Read the model definition and answer for the solid it produces. Units are mm, in the model's axes. Face numbers are marked on the shaded views. A direction names the side the tool comes from. Give positions to 0.01 mm unless a question says otherwise; leave off trailing zeros. Write each loop counter-clockwise with the first axis right and the second up, starting at its lowest first coordinate (ties: lowest second). Pieces come first, ordered by that corner, then holes. Notation, with made-up numbers: (-5, 43) -> (28, 43) arc R9 cw to (28, 49) -> close; hole circle Ø3 at (-32, 56.5). An arc over 180 degrees is marked (long way). Write item = value, one per line.
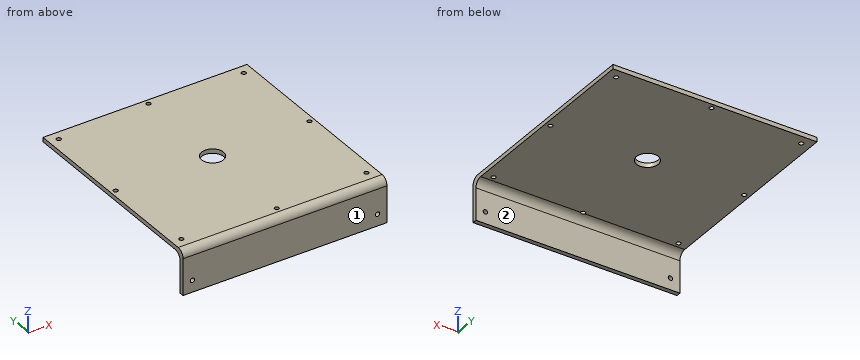
from build123d import *

# Parameters (mm, degrees)
SKICA1_W                 = 140
SKICA1_H                 = 145
SKICA1_R                 = 1.5
P_IDAT_VYSUNUT_M1_DEPTH  = 3
SKICA2_W                 = 140
SKICA2_H                 = 30
P_IDAT_VYSUNUT_M2_DEPTH  = 3
SKICA3_R                 = 1.5
ODEBRAT_VYSUNUT_M1_DEPTH = 161.601992516
ZAOBLIT1_R               = 5
SKICA4_R                 = 7.5
SKICA4_R_2               = 1.5
ODEBRAT_VYSUNUT_M2_DEPTH = 106.148704224


with BuildPart() as part:
    # Skica1 → Přidat vysunutím1 (new body)
    with BuildSketch(Plane.XY):
        Rectangle(SKICA1_W, SKICA1_H)
        with Locations((-63.5, 66)):
            Circle(SKICA1_R, mode=Mode.SUBTRACT)
        with Locations((-66.5, 2.5)):
            Circle(SKICA1_R, mode=Mode.SUBTRACT)
        with Locations(Location((63.5, 66, 0), (0, 0, 180))):
            Circle(SKICA1_R, mode=Mode.SUBTRACT)
        with Locations(Location((66.5, 2.5, 0), (0, 0, 180))):
            Circle(SKICA1_R, mode=Mode.SUBTRACT)
        with Locations((63.5, -61)):
            Circle(SKICA1_R, mode=Mode.SUBTRACT)
        with Locations(Location((-63.5, -61, 0), (0, 0, 180))):
            Circle(SKICA1_R, mode=Mode.SUBTRACT)
    extrude(amount=P_IDAT_VYSUNUT_M1_DEPTH)

    # Skica2 → Přidat vysunutím2 (add)
    with BuildSketch(Plane.XZ.offset(72.5)):
        with Locations((0, -12)):
            Rectangle(SKICA2_W, SKICA2_H)
    extrude(amount=-P_IDAT_VYSUNUT_M2_DEPTH)

    # Skica3 → Odebrat vysunutím1 (cut, through all)
    with BuildSketch(Plane(origin=(0, -69.5, 0), x_dir=(1, 0, 0), z_dir=(0, 1, 0))):
        with Locations(Location((-63.5, 19, 0), (0, 0, 270))):
            Circle(SKICA3_R)
        with Locations(Location((63.5, 19, 0), (0, 0, 90))):
            Circle(SKICA3_R)
    extrude(amount=-ODEBRAT_VYSUNUT_M1_DEPTH, mode=Mode.SUBTRACT)

    # Zaoblit1
    zaoblit1_edges = [part.edges().sort_by_distance(p)[0] for p in [
        (0, -72.5, 3),
        (0, -69.5, 0),
    ]]
    fillet(zaoblit1_edges, radius=ZAOBLIT1_R)

    # Skica4 → Odebrat vysunutím2 (cut, through all)
    with BuildSketch(Plane.XY.offset(3)):
        with Locations((0, 2.5)):
            Circle(SKICA4_R)
        with Locations((0, 69)):
            Circle(SKICA4_R_2)
        with Locations(Location((0, -64, 0), (0, 0, 340.528779366))):
            Circle(SKICA4_R_2)
    extrude(amount=-ODEBRAT_VYSUNUT_M2_DEPTH, mode=Mode.SUBTRACT)


solid = part.part
(1) The part is cut by section B-B on x = -4.5. Determine the outline of the cut face in (y, z), plus the area to 3 significant figures.
Checks:
outline = (-72.5, -27) -> (-69.5, -27) -> (-69.5, -5) arc R5 cw to (-64.5, 0) -> (-3.5, 0) -> (-3.5, 3) -> (-67.5, 3) arc R5 ccw to (-72.5, -2) -> close; (8.5, 0) -> (72.5, 0) -> (72.5, 3) -> (8.5, 3) -> close
area = 480 mm²
(2) A tool of negligible diameter and unlimited length cuts with its end or side. For the marked faces 1 and 2, from which of +Z, -Z, +X, -X, +Y, -Y can it reach the whole face along a straight path? Write none if from no direction.
Checks:
face_1 = +Z, -Z, +X, -X, -Y
face_2 = -Z, +X, -X, +Y
(3) Consider L1, parallel to X at y = 66, z = 1; L2, parallel to Y at x = -63, z = 2; L3, parallel to Y at x = 0, z = 1. Determine where each line is inside the solid, lowest interval first.
Checks:
L1 = -70 to -65, -62 to 62, 65 to 70
L2 = -70.5 to -62.41, -59.59 to 64.59, 67.41 to 72.5
L3 = -71.5 to -65.5, -62.5 to -5, 10 to 67.5, 70.5 to 72.5
(4) The part is cut by section D-D on y = 36. Determine the outline of the cut face in (x, z), plus the area to 3 significant figures.
Checks:
outline = (-70, 0) -> (70, 0) -> (70, 3) -> (-70, 3) -> close
area = 420 mm²
(5) Given P1, Ø4, axis at x = -63.5, z = -19, coming from the -Y side; P2, Ø3.5, axis at x = -63.5, y = 66, coming from the -Z side; P3, Ø2.5, axis at x = 63.5, y = 66, coming from the +Z side; P4, Ø6.5, axis at x = 30, z = -18, coming from the +Y side, each flat-ended and moving along its own axis, determine where each tip first touches the part or whether it passes through.
Checks:
P1 = -72.5
P2 = 0
P3 = through
P4 = -69.5
(6) The part is cut by section A-A on y = 7. Determine the outline of the cut face in (x, z), plus the area to 3 significant figures.
Checks:
outline = (-70, 0) -> (-6, 0) -> (-6, 3) -> (-70, 3) -> close; (6, 0) -> (70, 0) -> (70, 3) -> (6, 3) -> close
area = 384 mm²
(7) The part is cut by section C-C on z = -11.5. Determine the outline of the cut face in (x, y), plus the area to 3 significant figures.
Checks:
outline = (-70, -72.5) -> (70, -72.5) -> (70, -69.5) -> (-70, -69.5) -> close
area = 420 mm²
